Part print with two shaded views. Sizes in mm from the minimum x, y, z corner. Give positions to 0.01 mm unless a question says otherwise; leave off trailing zeros. Write each loop counter-clockwise with the first axis right and the second up, starting at its lowest first coordinate (ties: lowest second). Pieces come first, ordered by that corner, then holes.
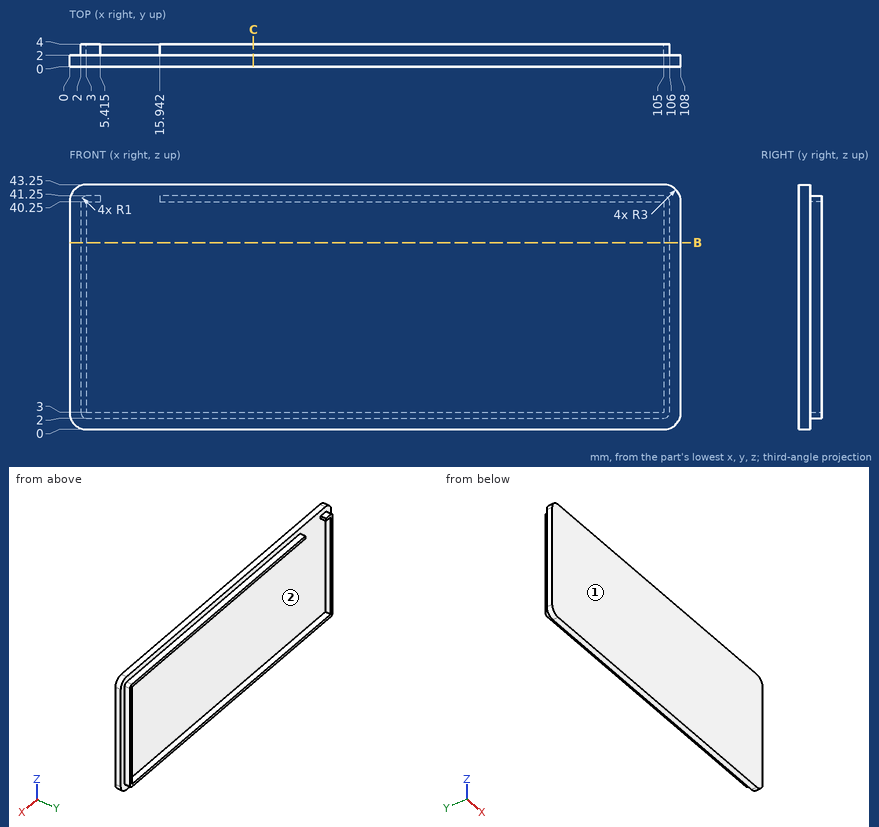
(1) Mould opens along X. For the marked faces 1 and 2 say: +X half, -X half, draft (parallel to the pull), parting line (faces both ways), or undercut.
(2) Drop flat-ended pins along their axis: pin 1 (0.8 mm diameter, centred on y = 2.5, z = 41, fed in from -X); pin 2 (10 mm diameter, centred on x = 48, z = 21.5, fed in from +Y); pin 3 (1.6 mm diameter, centred on x = 65.5, y = 3.5, fed in from -Z). Give the stop position or say it passes through.
(3) Saw through at B-B, the plane z = 33. List the corners of the cut face in (x, y), plus the area to 3 significant figures.
(4) Saw through at C-C, the plane x = 32.5. List the corners of the cut face in (y, z).
(5) Probe line 1 (X direction, y = 2.9, z = 22); line 2 (Z direction, x = 90.5, y = 3.35); line 3 (Y direction, x = 14, z = 15). List the from-to ranges inside material, lowest first.
Computed values:
1. face 1: draft
1. face 2: undercut
2. pin 1: stops at x = 2.06
2. pin 2: stops at y = 2
2. pin 3: stops at z = 2
3. outline: (0, 0) - (108, 0) - (108, 2) - (106, 2) - (106, 4) - (105, 4) - (105, 2) - (3, 2) - (3, 4) - (2, 4) - (2, 2) - (0, 2) - close
3. area: 220 mm2
4. outline: (0, 0) - (2, 0) - (2, 2) - (4, 2) - (4, 3) - (2, 3) - (2, 40.25) - (4, 40.25) - (4, 41.25) - (2, 41.25) - (2, 43.25) - (0, 43.25) - close
5. line 1: x = 2 to 3, 105 to 106
5. line 2: z = 2 to 3, 40.25 to 41.25
5. line 3: y = 0 to 2
